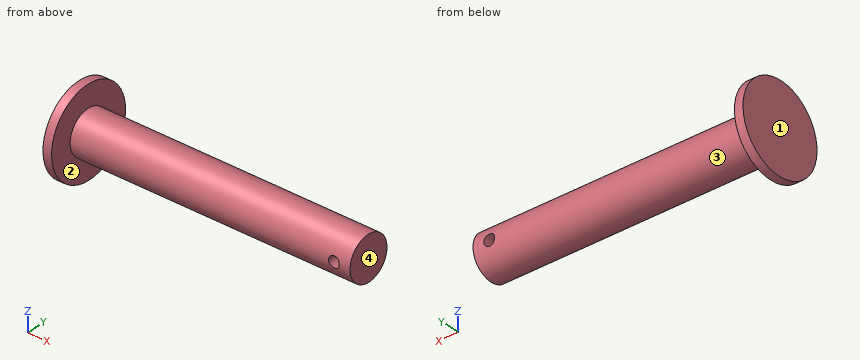
```python
from build123d import *

# Parameters (mm, degrees)
SKETCH1_R           = 12.7
BOSS_EXTRUDE1_DEPTH = 2.54
SKETCH2_R           = 6.35
BOSS_EXTRUDE2_DEPTH = 82.55
SKETCH3_R           = 1.5875
CUT_EXTRUDE1_DEPTH  = 12.7


with BuildPart() as part:
    # Sketch1 → Boss-Extrude1 (new body)
    with BuildSketch(Plane(origin=(0, 0, 0), x_dir=(0, 0, -1), z_dir=(1, 0, 0))):
        Circle(SKETCH1_R)
    extrude(amount=BOSS_EXTRUDE1_DEPTH)

    # Sketch2 → Boss-Extrude2 (add)
    with BuildSketch(Plane(origin=(2.54, 0, 0), x_dir=(0, 0, -1), z_dir=(1, 0, 0))):
        Circle(SKETCH2_R)
    extrude(amount=BOSS_EXTRUDE2_DEPTH)

    # Sketch3 → Cut-Extrude1 (cut, symmetric)
    with BuildSketch(Plane(origin=(0, 0, 0), x_dir=(1, 0, 0), z_dir=(0, 1, 0))):
        with Locations((80.3275, 0)):
            Circle(SKETCH3_R)
    extrude(amount=CUT_EXTRUDE1_DEPTH, both=True, mode=Mode.SUBTRACT)


solid = part.part
```
Check sheet for the modelled part. Datum: model origin and axes. Units: mm. Face numbers are marked on the shaded views. A direction names the side the tool comes from. Coordinates: 2 decimals unless noted, no trailing zeros. Write each loop counter-clockwise with the first axis right and the second up, starting at its lowest first coordinate (ties: lowest second). Pieces come first, ordered by that corner, then holes. Notation, with made-up numbers: (84.25, -3.5) -> (111.25, -3.5) arc R32 ccw to (111.25, 31.5) -> close; hole circle Ø9 at (89, 19). An arc over 180 degrees is marked (long way). Use a Markdown table: item, result.
1. Sectioned sample at D-D (z = -9.25). Enter the section's corners in (x, y), plus the area to 3 significant figures.
Reported:
| item | result |
|---|---|
| outline | (0, -8.7) -> (2.54, -8.7) -> (2.54, 8.7) -> (0, 8.7) -> close |
| area | 44.2 mm2 |
2. Tool access check on the marked faces 1 and 2. Record the directions out of +Z, -Z, +X, -X, +Y, -Y that give a thin tool (end or side, any length) a straight path to the whole face; none if there is none.
Reported:
| item | result |
|---|---|
| face 1 | +Z, -Z, -X, +Y, -Y |
| face 2 | +X |
3. Go/stop test with flat-tipped pins: pin 1 Ø3 at (x, z) = (63, 6) entering from +Y; pin 2 Ø3 at (x, z) = (76, 2.5) entering from -Y; pin 3 Ø5 at (x, y) = (37.5, -6) entering from +Z; pin 4 Ø5 at (x, y) = (32, -10) entering from +Z. Record where each tip stops, or that it passes through.
Reported:
| item | result |
|---|---|
| pin 1 | stops at y = 4.48 |
| pin 2 | stops at y = -6.27 |
| pin 3 | stops at z = 5.3 |
| pin 4 | passes through |
4. Sectioned sample at A-A (z = 0). Enter the section's corners in (x, y) (3 decimals), plus the area to 3 significant figures.
Reported:
| item | result |
|---|---|
| outline | (0, -12.7) -> (2.54, -12.7) -> (2.54, -6.35) -> (78.74, -6.35) -> (78.74, 6.35) -> (2.54, 6.35) -> (2.54, 12.7) -> (0, 12.7) -> close; (81.915, -6.35) -> (85.09, -6.35) -> (85.09, 6.35) -> (81.915, 6.35) -> close |
| area | 1,070 mm2 |
5. Sectioned sample at C-C (x = 17.5). Enter the section's corners in (y, z).
Reported:
| item | result |
|---|---|
| outline | circle Ø12.7 at (0, 0) |
6. Scan lines: line 1 along X through (y, z) = (1.5, 0) (3 decimals); line 2 along X through (y, z) = (-7, -2.25); line 3 along Z through (x, y) = (79, -3.5). Record each from-to range of solid material in increasing order.
Reported:
| item | result |
|---|---|
| line 1 | x = 0 to 78.74, 81.915 to 85.09 |
| line 2 | x = 0 to 2.54 |
| line 3 | z = -5.3 to -0.87, 0.87 to 5.3 |
7. Release check for a two-part mould opening along Z. For the marked faces 3 and 4 record: pulls with the +Z half, pulls with the -Z half, needs draft (parallel to the pull), parting line crosses it, or undercut.
Reported:
| item | result |
|---|---|
| face 3 | parting line crosses it |
| face 4 | needs draft |
